from build123d import *

# Parameters (mm, degrees)
F0_R      = 2
F1_DEPTH  = 7
F2_R      = 5
F3_W      = 3.4330971539
F3_H      = 4.5472582311
F4_DEPTH  = 25
F5_R      = 2.25
F6_DEPTH  = 25
F7_R      = 2.25
F7_R_2    = 0.82
F8_DEPTH  = 2.5
F9_DEPTH  = 4.5
F10_DEPTH = 2


with BuildPart() as f1:
    # F0 (on Top) → F1 (new body)
    with BuildSketch(Plane.XY):
        with BuildLine():
            Line((-23.9209998254, 63.5463201136), (-21.9209998254, 63.5463201136))
            Line((-21.9209998254, 63.5463201136), (-21.9209998254, 71.0463201136))
            Line((-21.9209998254, 71.0463201136), (-29.4209998254, 71.0463201136))
            Line((-29.4209998254, 71.0463201136), (-29.4209998254, 69.0463201136))
            Line((-29.4209998254, 69.0463201136), (-29.4209998254, 65.5539904986))
            ThreePointArc((-29.4209998254, 65.5539904986), (-28.3799049656, 64.5874149733), (-27.4133294404, 63.5463201136))
            Line((-27.4133294404, 63.5463201136), (-23.9209998254, 63.5463201136))
        make_face()
        with Locations((-25.8659998254, 66.9521987438)):
            Circle(F0_R, mode=Mode.SUBTRACT)
        with BuildLine():
            Line((-29.4209998254, 65.5539904986), (-29.4209998254, 69.0463201136))
            Line((-29.4209998254, 69.0463201136), (-35.3847547259, 69.0463201136))
            ThreePointArc((-35.3847547259, 69.0463201136), (-32.244029824, 67.5714147152), (-29.4209998254, 65.5539904986))
        make_face()
        with BuildLine():
            Line((-29.4209998254, 69.0463201136), (-29.4209998254, 71.0463201136))
            Line((-29.4209998254, 71.0463201136), (-54.4209998254, 71.0463201136))
            Line((-54.4209998254, 71.0463201136), (-54.4209998254, 69.0463201136))
            Line((-54.4209998254, 69.0463201136), (-48.4572449248, 69.0463201136))
            ThreePointArc((-48.4572449248, 69.0463201136), (-41.9209998254, 70.1963201136), (-35.3847547259, 69.0463201136))
            Line((-35.3847547259, 69.0463201136), (-29.4209998254, 69.0463201136))
        make_face()
        with BuildLine():
            Line((-48.4572449248, 69.0463201136), (-54.4209998254, 69.0463201136))
            Line((-54.4209998254, 69.0463201136), (-54.4209998254, 65.5539904986))
            ThreePointArc((-54.4209998254, 65.5539904986), (-51.5979698267, 67.5714147152), (-48.4572449248, 69.0463201136))
        make_face()
        with BuildLine():
            Line((-61.9209998254, 71.0463201136), (-61.9209998254, 63.5463201136))
            Line((-61.9209998254, 63.5463201136), (-59.9209998254, 63.5463201136))
            Line((-59.9209998254, 63.5463201136), (-56.4286702104, 63.5463201136))
            ThreePointArc((-56.4286702104, 63.5463201136), (-55.4620946851, 64.5874149733), (-54.4209998254, 65.5539904986))
            Line((-54.4209998254, 65.5539904986), (-54.4209998254, 69.0463201136))
            Line((-54.4209998254, 69.0463201136), (-54.4209998254, 71.0463201136))
            Line((-54.4209998254, 71.0463201136), (-61.9209998254, 71.0463201136))
        make_face()
        with Locations((-57.9759998254, 66.9521987438)):
            Circle(F0_R, mode=Mode.SUBTRACT)
        with BuildLine():
            Line((-56.4286702104, 63.5463201136), (-59.9209998254, 63.5463201136))
            Line((-59.9209998254, 63.5463201136), (-59.9209998254, 57.582565213))
            ThreePointArc((-59.9209998254, 57.582565213), (-58.446094427, 60.7232901149), (-56.4286702104, 63.5463201136))
        make_face()
        with BuildLine():
            Line((-61.9209998254, 63.5463201136), (-61.9209998254, 38.5463201136))
            Line((-61.9209998254, 38.5463201136), (-59.9209998254, 38.5463201136))
            Line((-59.9209998254, 38.5463201136), (-59.9209998254, 44.5100750141))
            ThreePointArc((-59.9209998254, 44.5100750141), (-61.0709998254, 51.0463201136), (-59.9209998254, 57.582565213))
            Line((-59.9209998254, 57.582565213), (-59.9209998254, 63.5463201136))
            Line((-59.9209998254, 63.5463201136), (-61.9209998254, 63.5463201136))
        make_face()
        with BuildLine():
            Line((-59.9209998254, 44.5100750141), (-59.9209998254, 38.5463201136))
            Line((-59.9209998254, 38.5463201136), (-56.4286702104, 38.5463201136))
            ThreePointArc((-56.4286702104, 38.5463201136), (-58.446094427, 41.3693501123), (-59.9209998254, 44.5100750141))
        make_face()
        with BuildLine():
            Line((-61.9209998254, 31.0463201136), (-54.4209998254, 31.0463201136))
            Line((-54.4209998254, 31.0463201136), (-54.4209998254, 33.0463201136))
            Line((-54.4209998254, 33.0463201136), (-54.4209998254, 36.5386497286))
            ThreePointArc((-54.4209998254, 36.5386497286), (-55.4620946851, 37.5052252539), (-56.4286702104, 38.5463201136))
            Line((-56.4286702104, 38.5463201136), (-59.9209998254, 38.5463201136))
            Line((-59.9209998254, 38.5463201136), (-61.9209998254, 38.5463201136))
            Line((-61.9209998254, 38.5463201136), (-61.9209998254, 31.0463201136))
        make_face()
        with Locations((-57.9759998254, 35.1404414833)):
            Circle(F0_R, mode=Mode.SUBTRACT)
        with BuildLine():
            Line((-54.4209998254, 36.5386497286), (-54.4209998254, 33.0463201136))
            Line((-54.4209998254, 33.0463201136), (-48.4572449248, 33.0463201136))
            ThreePointArc((-48.4572449248, 33.0463201136), (-51.5979698267, 34.5212255119), (-54.4209998254, 36.5386497286))
        make_face()
        with BuildLine():
            Line((-54.4209998254, 31.0463201136), (-29.4209998254, 31.0463201136))
            Line((-29.4209998254, 31.0463201136), (-29.4209998254, 33.0463201136))
            Line((-29.4209998254, 33.0463201136), (-35.3847547259, 33.0463201136))
            ThreePointArc((-35.3847547259, 33.0463201136), (-41.9209998254, 31.8963201136), (-48.4572449248, 33.0463201136))
            Line((-48.4572449248, 33.0463201136), (-54.4209998254, 33.0463201136))
            Line((-54.4209998254, 33.0463201136), (-54.4209998254, 31.0463201136))
        make_face()
        with BuildLine():
            Line((-35.3847547259, 33.0463201136), (-29.4209998254, 33.0463201136))
            Line((-29.4209998254, 33.0463201136), (-29.4209998254, 36.5386497286))
            ThreePointArc((-29.4209998254, 36.5386497286), (-32.244029824, 34.5212255119), (-35.3847547259, 33.0463201136))
        make_face()
        with BuildLine():
            Line((-29.4209998254, 31.0463201136), (-21.9209998254, 31.0463201136))
            Line((-21.9209998254, 31.0463201136), (-21.9209998254, 38.5463201136))
            Line((-21.9209998254, 38.5463201136), (-23.9209998254, 38.5463201136))
            Line((-23.9209998254, 38.5463201136), (-27.4133294404, 38.5463201136))
            ThreePointArc((-27.4133294404, 38.5463201136), (-28.3799049656, 37.5052252539), (-29.4209998254, 36.5386497286))
            Line((-29.4209998254, 36.5386497286), (-29.4209998254, 33.0463201136))
            Line((-29.4209998254, 33.0463201136), (-29.4209998254, 31.0463201136))
        make_face()
        with Locations((-25.8659998254, 35.1404414833)):
            Circle(F0_R, mode=Mode.SUBTRACT)
        with BuildLine():
            Line((-27.4133294404, 38.5463201136), (-23.9209998254, 38.5463201136))
            Line((-23.9209998254, 38.5463201136), (-23.9209998254, 44.5100750141))
            ThreePointArc((-23.9209998254, 44.5100750141), (-25.3959052237, 41.3693501123), (-27.4133294404, 38.5463201136))
        make_face()
        with BuildLine():
            Line((-23.9209998254, 38.5463201136), (-21.9209998254, 38.5463201136))
            Line((-21.9209998254, 38.5463201136), (-21.9209998254, 63.5463201136))
            Line((-21.9209998254, 63.5463201136), (-23.9209998254, 63.5463201136))
            Line((-23.9209998254, 63.5463201136), (-23.9209998254, 57.582565213))
            ThreePointArc((-23.9209998254, 57.582565213), (-23.0606909732, 54.3646404718), (-22.7709998254, 51.0463201136))
            ThreePointArc((-22.7709998254, 51.0463201136), (-23.0606909732, 47.7279997553), (-23.9209998254, 44.5100750141))
            Line((-23.9209998254, 44.5100750141), (-23.9209998254, 38.5463201136))
        make_face()
        with BuildLine():
            Line((-23.9209998254, 57.582565213), (-23.9209998254, 63.5463201136))
            Line((-23.9209998254, 63.5463201136), (-27.4133294404, 63.5463201136))
            ThreePointArc((-27.4133294404, 63.5463201136), (-25.3959052237, 60.7232901149), (-23.9209998254, 57.582565213))
        make_face()
    extrude(amount=F1_DEPTH)

    # F2
    f2_edges = [f1.edges().sort_by_distance(p)[0] for p in [
        (-21.921, 31.04632, 3.5),
        (-61.921, 31.04632, 3.5),
        (-21.921, 71.04632, 3.5),
        (-61.921, 71.04632, 3.5),
    ]]
    fillet(f2_edges, radius=F2_R)

    # F3 (on face) → F4 (cut)
    with BuildSketch(Plane.XY.offset(7)):
        with Locations((-50.7930722088, 68.772690998)):
            Rectangle(F3_W, F3_H)
    extrude(amount=-F4_DEPTH, mode=Mode.SUBTRACT)

    # F5 (on face) → F6 (cut)
    with BuildSketch(Plane.XY.offset(7)):
        with Locations((-57.9759998254, 66.9521987438)):
            Circle(F5_R)
        with Locations((-25.8659998254, 66.9521987438)):
            Circle(F5_R)
        with Locations((-25.8659998254, 35.1404414833)):
            Circle(F5_R)
        with Locations((-57.9759998254, 35.1404414833)):
            Circle(F5_R)
    extrude(amount=-F6_DEPTH, mode=Mode.SUBTRACT)

    # F7 (on face) → F8 (join)
    with BuildSketch(Plane(origin=(0, 0, 0), x_dir=(1, 0, 0), z_dir=(0, 0, -1))):
        with Locations((-25.8659998254, -66.9521987438)):
            Circle(F7_R)
        with Locations((-25.8659998254, -66.9521987438)):
            Circle(F7_R_2, mode=Mode.SUBTRACT)
        with Locations((-57.9759998254, -66.9521987438)):
            Circle(F7_R)
        with Locations((-57.9759998254, -66.9521987438)):
            Circle(F7_R_2, mode=Mode.SUBTRACT)
        with Locations((-57.9759998254, -35.1404414833)):
            Circle(F7_R)
        with Locations((-57.9759998254, -35.1404414833)):
            Circle(F7_R_2, mode=Mode.SUBTRACT)
        with Locations((-25.8659998254, -35.1404414833)):
            Circle(F7_R)
        with Locations((-25.8659998254, -35.1404414833)):
            Circle(F7_R_2, mode=Mode.SUBTRACT)
    extrude(amount=-F8_DEPTH)

    # F9 (add): faces of the model
    f9_faces = [f1.faces().sort_by_distance(p)[0] for p in [
        (-28.0523602151, 66.9521987438, 2.5),
        (-60.1623602151, 35.1404414833, 2.5),
    ]]
    extrude(f9_faces, amount=F9_DEPTH)

    # F10 (add): faces of the model
    f10_faces = [f1.faces().sort_by_distance(p)[0] for p in [
        (-60.1623602151, 66.9521987438, 2.5),
        (-28.0523602151, 35.1404414833, 2.5),
    ]]
    extrude(f10_faces, amount=F10_DEPTH)


solid = f1.part
Read the model definition and answer for the solid it produces. Units are mm, in the model's axes. A direction names the side the tool comes from. Round coordinates to 2 decimals unless told otherwise and drop trailing zeros. Loops run counter-clockwise (first coordinate to the right, second up) from the corner with the lowest first, then second, coordinate; pieces in that order, holes last.
Q1. Each of these flat-tipped pins is pushed along its axis until it touches: pin 1 (2 mm diameter, centred on y = 35, z = 2, fed in from +X); pin 2 (1.3 mm diameter, centred on x = -58.5, y = 66.5, fed in from +Z); pin 3 (2 mm diameter, centred on y = 68.5, z = 4, fed in from +X); pin 4 (1.8 mm diameter, centred on y = 70, z = 4.5, fed in from -X). Where does it stop, or does it pass through?
Q2. Consider probe 1 along X at (y, z) = (67, 0.5); probe 2 along Y at (x, z) = (-58.5, 3.5); probe 3 along X at (y, z) = (40, 6). Determine where each line is inside the solid, lowest interval first.
Q3. Determine the mould class of faces 4 (the face through (-25.973, 34.327, 2.218)), 5 (the face through (-57, 67, 4.5)), 6 (the face through (-60.42, 69.62, 3.55)), 7 (the face through (-23.425, 32.472, 3.549)) for opening direction Y: released by +Y, released by -Y, zero draft, split by the parting line, or undercut.
Q4. Which of the six approach directions +Z, -Z, +X, -X, +Y, -Y give full straight-line access (tool end or side, diameter ignored) to faces 1 (the face through (-49.077, 70, 4)), 2 (the face through (-25.9, 36.11, 4.5)), 3 (the face through (-61.921, 51, 3))?
Q5. Section A-A on y = 62.5 is taken. Write down the section's boundary in (x, z), and give its area (3 significant figures).
Q6. Section B-B on x = -26 is taken. Write down the section's boundary in (y, z), and give its area (4 significant figures).
Q7. Section D-D on x = -38 is taken. Write down the section's boundary in (y, z), and give its area (3 significant figures).
Q8. Section C-C on z = 1.25 is taken. Write down the section's boundary in (x, y).
Output:
1. pin 1: stops at x = -21.92
1. pin 2: stops at z = 4.5
1. pin 3: stops at x = -22.14
1. pin 4: stops at x = -60.88
2. probe 1: x = -61.83 to -58.79, -57.16 to -52.51, -31.33 to -26.68, -25.05 to -22.01
2. probe 2: y = 31.3 to 34.51, 35.77 to 41.46, 60.63 to 66.32, 67.58 to 70.79
2. probe 3: x = -61.92 to -57.56, -26.28 to -21.92
3. face 4: undercut
3. face 5: undercut
3. face 6: released by +Y
3. face 7: released by -Y
4. face 1: +Z, -Z, +Y
4. face 2: +Z
4. face 3: +Z, -Z, -X, +Y, -Y
5. outline: (-61.92, 0) - (-57.27, 0) - (-57.27, 7) - (-61.92, 7) - close; (-26.57, 0) - (-21.92, 0) - (-21.92, 7) - (-26.57, 7) - close
5. area: 65.1 mm2
6. outline: (31.13, 0) - (34.33, 0) - (34.33, 4.5) - (32.89, 4.5) - (32.89, 7) - (31.13, 7) - close; (35.95, 0) - (40.4, 0) - (40.4, 7) - (37.39, 7) - (37.39, 4.5) - (35.95, 4.5) - close; (61.69, 0) - (66.14, 0) - (66.14, 7) - (61.69, 7) - close; (67.76, 0) - (70.96, 0) - (70.96, 7) - (67.76, 7) - close
6. area: 100.0 mm2
7. outline: (31.05, 0) - (32.3, 0) - (32.3, 7) - (31.05, 7) - close; (69.79, 0) - (71.05, 0) - (71.05, 7) - (69.79, 7) - close
7. area: 17.6 mm2
8. outline: (-61.92, 36.05) arc R5 ccw to (-56.92, 31.05) - (-26.92, 31.05) arc R5 ccw to (-21.92, 36.05) - (-21.92, 66.05) arc R5 ccw to (-26.92, 71.05) - (-49.08, 71.05) - (-49.08, 68.81) arc R19.15 cw (long way) to (-52.51, 67) - (-52.51, 71.05) - (-56.92, 71.05) arc R5 ccw to (-61.92, 66.05) - close; hole circle Ø1.64 at (-57.98, 35.14); hole circle Ø1.64 at (-57.98, 66.95); hole circle Ø1.64 at (-25.87, 35.14); hole circle Ø1.64 at (-25.87, 66.95)
